Input: part model. Units: mm. Frame: model coordinates. Face numbers are marked on the shaded views. A direction names the side the tool comes from. Coordinates: 2 decimals unless noted, no trailing zeros. Write each loop counter-clockwise with the first axis right and the second up, starting at its lowest first coordinate (ties: lowest second). Pieces come first, ordered by that corner, then holes. Notation, with made-up numbers: (-14.5, 64.25) - (-6.5, 64.25) arc R18 cw to (-6.5, 80.25) - close; hole circle Ø3 at (17, 27.25). An arc over 180 degrees is marked (long way). Use a Markdown table: item, result. Add a question column.
Q1. Pin query (flat end, axial travel): P1, Ø6.5, axis at y = -5.5, z = -11, coming from the -X side; P2, Ø10, axis at x = 23, y = -9, coming from the +Z side; P3, Ø10.5, axis at y = -8.5, z = -10, coming from the +X side; P4, Ø1, axis at y = -1.5, z = -13.5, coming from the +X side. Return the tip coordinate at first contact, or that it passes through.
Q2. Material intervals for probe 1 along Z at (x, y) = (41.65, -8.5); probe 2 along Z at (x, y) = (-36.5, -2.5); probe 3 along Y at (x, z) = (-42.6, -10), sorted ascending. Write a range as from..to.
Q3. Section query A-A (y = -10). Return the cut outline in (x, z), then the cut area to 3 significant figures.
Q4. Section query D-D (x = 27). Return the cut outline in (y, z).
Q5. Section query C-C (x = -10). Return the cut outline in (y, z).
Q6. Set-up query: the marked faces 1 and 2. Return all of +Z, -Z, +X, -X, +Y, -Y with unobstructed straight access to the full face (end or side cutting, diameter ignored); none if empty.
Q7. Mould query, pull axis Z, two halves, no side actions, for the marked faces 3 and 4. Classes: released by +Z, released by -Z, zero draft, split by the parting line, or undercut.
Q8. Section query B-B (y = 9). Return the cut outline in (x, z), then the cut area to 3 significant figures.
from build123d import *

# Parameters (mm, degrees)
BOSS_EXTRUDE1_DEPTH = 20
SKETCH2_W           = 5
SKETCH2_H           = 5
BOSS_EXTRUDE2_DEPTH = 20
SKETCH4_W           = 20
SKETCH4_H           = 17
SKETCH3_W           = 19.999551015
SKETCH3_H           = 17
SKETCH6_W           = 20
SKETCH6_H           = 17
SKETCH5_W           = 20
SKETCH5_H           = 2
SKETCH7_R           = 2.75
CUT_EXTRUDE1_DEPTH  = 11.47488838
SKETCH8_R           = 6.5
CUT_EXTRUDE2_DEPTH  = 30


with BuildPart() as part:
    # Sketch1 → Boss-Extrude1 (new body)
    with BuildSketch(Plane(origin=(0, 0, 0), x_dir=(1, 0, 0), z_dir=(0, 1, 0))):
        Polygon((-45.74, 0), (-45.315821408, 20), (45.315821408, 20), (45.74, 0), align=None)
    extrude(amount=BOSS_EXTRUDE1_DEPTH)

    # Sketch2 → Boss-Extrude2 (add)
    with BuildSketch(Plane(origin=(0, 20, 0), x_dir=(1, 0, 0), z_dir=(0, 1, 0))):
        with Locations((47.97488838, 10)):
            Rectangle(SKETCH2_W, SKETCH2_H)
        with Locations((-47.97488838, 10)):
            Rectangle(SKETCH2_W, SKETCH2_H)
    extrude(amount=-BOSS_EXTRUDE2_DEPTH)

    # Sketch4 → Loft1 section 0
    with BuildSketch(Plane(origin=(-40, 0, 0), x_dir=(0, 0, -1), z_dir=(1, 0, 0))):
        with Locations((10, -8.5)):
            Rectangle(SKETCH4_W, SKETCH4_H)
    # Sketch3 → Loft1 section 1
    with BuildSketch(Plane(origin=(-45.719434544, 0, -0.969660269), x_dir=(-0.021204161, 0, 0.999775167), z_dir=(-0.999775167, 0, -0.021204161))):
        with Locations((-9.034843843, -8.5)):
            Rectangle(SKETCH3_W, SKETCH3_H)
    loft1 = loft()

    # Sketch6 → Loft3 section 0
    with BuildSketch(Plane(origin=(-40, 0, 0), x_dir=(0, 0, -1), z_dir=(1, 0, 0))):
        with Locations((10, -8.5)):
            Rectangle(SKETCH6_W, SKETCH6_H)
    # Sketch5 → Loft3 section 1
    with BuildSketch(Plane(origin=(-20, 0, 0), x_dir=(0, 0, -1), z_dir=(1, 0, 0))):
        with Locations((10, -1)):
            Rectangle(SKETCH5_W, SKETCH5_H)
    loft3 = loft()

    # Sketch7 → Cut-Extrude1 (cut, through all)
    with BuildSketch(Plane(origin=(-40, 0, 0), x_dir=(0, 0, -1), z_dir=(1, 0, 0))):
        with Locations((10, -8.5)):
            Circle(SKETCH7_R)
    cut_extrude1 = extrude(amount=-CUT_EXTRUDE1_DEPTH, mode=Mode.SUBTRACT)

    # Sketch8 → Cut-Extrude2 (cut)
    with BuildSketch(Plane(origin=(-40, 0, 0), x_dir=(0, 0, -1), z_dir=(1, 0, 0))):
        with Locations((10, -8.5)):
            Circle(SKETCH8_R)
    cut_extrude2 = extrude(amount=CUT_EXTRUDE2_DEPTH, mode=Mode.SUBTRACT)

    # Mirror1: Loft1, Loft3, Cut-Extrude1, Cut-Extrude2 across plane
    add(loft1.mirror(Plane(origin=(0, 0, 0), x_dir=(0, 0, 1), z_dir=(1, 0, 0))))
    add(loft3.mirror(Plane(origin=(0, 0, 0), x_dir=(0, 0, 1), z_dir=(1, 0, 0))))
    add(cut_extrude1.mirror(Plane(origin=(0, 0, 0), x_dir=(0, 0, 1), z_dir=(1, 0, 0))), mode=Mode.SUBTRACT)
    add(cut_extrude2.mirror(Plane(origin=(0, 0, 0), x_dir=(0, 0, 1), z_dir=(1, 0, 0))), mode=Mode.SUBTRACT)


solid = part.part
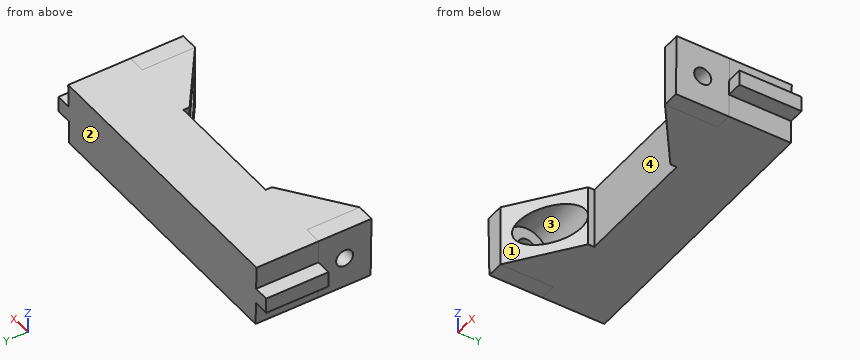
Values follow:
| question | item | result |
|---|---|---|
| 1 | P1 | x = -45.58 |
| 1 | P2 | z = 0 |
| 1 | P3 | x = 45.64 |
| 1 | P4 | x = 45.46 |
| 2 | probe 1 | -20..-12.75, -7.25..0 |
| 2 | probe 2 | -20..-12.5, -7.5..0 |
| 2 | probe 3 | -17..-11.25, -5.75..20 |
| 3 | outline | (-45.74, 0) - (-45.58, -7.7) - (-40, -7.7) - (-40, -3.68) - (-30.67, -3.68) - (-30.67, 0) - (-40, 0) - close; (-45.48, -12.3) - (-45.32, -20) - (-30.67, -20) - (-30.67, -16.32) - (-40, -16.32) - (-40, -12.3) - close; (30.67, -20) - (45.32, -20) - (45.48, -12.3) - (40, -12.3) - (40, -16.32) - (30.67, -16.32) - close; (30.67, -3.68) - (40, -3.68) - (40, -7.7) - (45.58, -7.7) - (45.74, 0) - (40, 0) - (30.67, 0) - close |
| 3 | area | 307 mm2 |
| 4 | outline | (-7.25, -20) - (20, -20) - (20, 0) - (-7.25, 0) - (-7.25, -3.62) arc R6.5 cw to (-7.25, -16.38) - close |
| 5 | outline | (0, -20) - (20, -20) - (20, 0) - (0, 0) - close |
| 6 | face 1 | +Z, -Z, -Y |
| 6 | face 2 | +Z, -Z, +X, -X, +Y |
| 7 | face 3 | undercut |
| 7 | face 4 | zero draft |
| 8 | outline | (-50.47, -12.5) - (-45.47, -12.5) - (-45.32, -20) - (45.32, -20) - (45.47, -12.5) - (50.47, -12.5) - (50.47, -7.5) - (45.58, -7.5) - (45.74, 0) - (-45.74, 0) - (-45.58, -7.5) - (-50.47, -7.5) - close |
| 8 | area | 1,870 mm2 |
